Autodesk Inventor part; units mm, degrees
ref_plane "YZ Plane" through (0, 0, 0) normal (1, 0, 0) x (0, 1, 0)
ref_plane "XZ Plane" through (0, 0, 0) normal (0, 1, 0) x (-1, 0, 0)
ref_plane "XY Plane" through (0, 0, 0) normal (0, 0, 1) x (1, 0, 0)
sketch "Esquisse1" plane through (0, 0, 0) normal (0, 1, 0) x (-1, 0, 0)
  line L0 (-7, 22.5) -> (7, 22.5)
  line L1 (9, 20.5) -> (9, -20.5)
  line L2 (7, -22.5) -> (-7, -22.5)
  line L3 (-9, -20.5) -> (-9, 20.5)
  line L4 (-9, 22.5) -> (9, -22.5) construction
  line L5 (9, 22.5) -> (-9, -22.5) construction
  line L6 (-5, -17.5) -> (5, -17.5) construction
  line L7 (5, -17.5) -> (5, 17.5) construction
  line L8 (5, 17.5) -> (-5, 17.5) construction
  line L9 (-5, 17.5) -> (-5, -17.5) construction
  line L10 (-5, -17.5) -> (5, 17.5) construction
  line L11 (5, -17.5) -> (-5, 17.5) construction
  arc A0 (9, 20.5) -> (7, 22.5) centre (7, 20.5) ccw
  arc A1 (-7, 22.5) -> (-9, 20.5) centre (-7, 20.5) ccw
  arc A2 (-9, -20.5) -> (-7, -22.5) centre (-7, -20.5) ccw
  arc A3 (7, -22.5) -> (9, -20.5) centre (7, -20.5) ccw
  point P0 (0, 0)
  dimension "d0" = 18
  dimension "d1" = 45
  dimension "d3" = 4
  dimension "d4" = 5
  dimension "d25" = 2
extrude "Extrusion1" add sketch "Esquisse1" against normal blind 8
hole "Perçage1" at (-5, 0, 17.5) at (5, 0, 17.5) at (5, 0, -17.5) at (-5, 0, -17.5) direction (0, -1, 0) diameter 4.2 end through all countersink diameter 9 countersink angle 90
sketch "Esquisse2" plane through (0, 0, 0) normal (0, 1, 0) x (1, 0, 0)
  line L0 (-9, -20.5) -> (-9, 20.5) construction
  line L1 (9, 13) -> (-9, 13) construction
  line L2 (-9, 13) -> (-9, -13) construction
  line L3 (-9, -13) -> (9, -13) construction
  line L4 (9, -13) -> (9, 13) construction
  line L5 (9, 13) -> (-9, -13) construction
  line L6 (-9, 13) -> (9, -13) construction
  line L7 (9, 7.5) -> (4.2, 7.5)
  line L8 (1.2, 4.5) -> (1.2, -4.5)
  line L9 (4.2, -7.5) -> (9, -7.5)
  line L10 (9, -7.5) -> (9, 7.5)
  arc A0 (1.2, -4.5) -> (4.2, -7.5) centre (4.2, -4.5) ccw
  arc A1 (4.2, 7.5) -> (1.2, 4.5) centre (4.2, 4.5) ccw
  line L11 (9, -13) -> (-9, -13)
  line L12 (-9, -9) -> (9, -9)
  line L13 (9, -9) -> (9, -13)
  line L14 (9, 13) -> (1.2, 13)
  line L15 (1.2, 13) -> (1.2, 9)
  line L16 (1.2, 9) -> (9, 9)
  line L17 (9, 9) -> (9, 13)
  line L18 (0, -22.5) -> (0, 22.5)
  line L19 (-7, -22.5) -> (7, -22.5) construction
  line L20 (7, 22.5) -> (-7, 22.5) construction
  line L21 (-9, -13) -> (-9, 13) construction
  line L22 (-9, 7.5) -> (-4.2, 7.5)
  line L23 (-1.2, 4.5) -> (-1.2, -4.5)
  line L24 (-4.2, -7.5) -> (-9, -7.5)
  line L25 (-9, -7.5) -> (-9, 7.5)
  arc A2 (-4.2, -7.5) -> (-1.2, -4.5) centre (-4.2, -4.5) ccw
  arc A3 (-1.2, 4.5) -> (-4.2, 7.5) centre (-4.2, 4.5) ccw
  line L26 (-9, -9) -> (-9, -13)
  line L27 (-9, 13) -> (-1.2, 13)
  line L28 (-1.2, 13) -> (-1.2, 9)
  line L29 (-1.2, 9) -> (-9, 9)
  line L30 (-9, 9) -> (-9, 13)
  point P0 (0, 0)
  point P1 (-9, -22.5)
  point P2 (-9, 22.5)
  dimension "d17" = 1.5
  dimension "d19" = 15
  dimension "d20" = 4
  dimension "d21" = 3
  dimension "d22" = 4
  dimension "d23" = 1.5
  dimension "d24" = 1.2
extrude "Extrusion2" add sketch "Esquisse2" along normal blind 10
properties part number "jonction de courroie"
Check sheet for the modelled part. Datum: model origin and axes. Units: mm. A direction names the side the tool comes from. Round coordinates to 2 decimals unless told otherwise and drop trailing zeros. Order: outer loops, then holes, each group sorted by start corner. A loop starts at its lowest first (then second) coordinate and runs counter-clockwise, first axis right, second up. Notation, with made-up numbers: (26.5, 64.25) -> (58.5, 64.25) arc R14 cw to (58.5, 79.25) -> close; hole circle Ø4 at (70.25, 47). An arc over 180 degrees is marked (long way). One line per item, written item: value. Start each with the question number.
Q1. Mould release check, pull along Z, two halves, no side actions. Record for faces 6 (the face through (5, 5, -9)), 7 (the face through (0, -4, 22.5)), 8 (the face through (-8.4, -3.94, -21.93)), 9 (the face through (-2.06, 4.93, 6.6)): pulls with the +Z half, pulls with the -Z half, needs draft (parallel to the pull), parting line crosses it, or undercut.
Q2. Cross-section at B-B (y = -6.25). Record the boundary of the cut face in (x, z).
Q3. Set-up check for faces 1 (the face through (0, 5, 13)), 2 (the face through (-2.1, 4.93, -6.64)), 3 (the face through (-5, 10, -11)), 4 (the face through (7, 5, 7.5)), 5 (the face through (9, -1, 0)): record each of +Z, -Z, +X, -X, +Y, -Y from which the full face is reachable in a straight line by a thin tool's end or side.
Q4. Gauge pin test, flat ends, axial feed: pin 1 Ø2.5 at (x, y) = (7, 4.5) entering from -Z; pin 2 Ø8 at (x, y) = (4.5, 6.5) entering from +Z; pin 3 Ø0.7 at (x, z) = (7, -14) entering from +Y. Record the tip position at first contact, or that the pin passes through.
Q5. Cross-section at A-A (z = -17.5). Record the boundary of the cut face in (x, y).
Q6. Thickness scan on line 1 (X direction, y = -5.7, z = 17.5); line 2 (Z direction, x = 7, y = 0.25); line 3 (Z direction, x = -5, y = -6.5). Record the ranges inside material, lowest first.
Q7. Cross-section at D-D (z = -9.5). Record the boundary of the cut face in (x, y).
Q8. Cross-section at C-C (y = 3.75). Record the boundary of the cut face in (x, z), and give its area (3 significant figures).
Completed:
1. face 6: undercut
1. face 7: pulls with the +Z half
1. face 8: pulls with the -Z half
1. face 9: undercut
2. outline: (-9, -20.5) arc R2 ccw to (-7, -22.5) -> (7, -22.5) arc R2 ccw to (9, -20.5) -> (9, 20.5) arc R2 ccw to (7, 22.5) -> (-7, 22.5) arc R2 ccw to (-9, 20.5) -> close; hole circle Ø4.2 at (-5, -17.5); hole circle Ø4.2 at (-5, 17.5); hole circle Ø4.2 at (5, -17.5); hole circle Ø4.2 at (5, 17.5)
3. face 1: +Z, +X, -X, +Y
3. face 2: +Y
3. face 3: +Z, -Z, +X, -X, +Y
3. face 4: +X, -X, +Y
3. face 5: +Z, -Z, +X, +Y, -Y
4. pin 1: stops at z = -13
4. pin 2: stops at z = 13
4. pin 3: stops at y = -0.12
5. outline: (-9, -8) -> (-7.1, -8) -> (-7.1, -2.4) -> (-9, -0.5) -> close; (-2.9, -8) -> (2.9, -8) -> (2.9, -2.4) -> (0.5, 0) -> (-0.5, 0) -> (-2.9, -2.4) -> close; (7.1, -8) -> (9, -8) -> (9, -0.5) -> (7.1, -2.4) -> close
6. line 1: x = -9 to -7.1, -2.9 to 2.9, 7.1 to 9
6. line 2: z = -13 to -9, -7.5 to 7.5, 9 to 13
6. line 3: z = -22.5 to -19.6, -15.4 to 15.4, 19.6 to 22.5
7. outline: (-9, -8) -> (9, -8) -> (9, 10) -> (1.2, 10) -> (1.2, 0) -> (-1.2, 0) -> (-1.2, 10) -> (-9, 10) -> close
8. outline: (-9, -13) -> (-1.2, -13) -> (-1.2, -9) -> (-9, -9) -> close; (-9, -7.5) -> (-4.2, -7.5) arc R3 ccw to (-1.2, -4.5) -> (-1.2, 4.5) arc R3 ccw to (-4.2, 7.5) -> (-9, 7.5) -> close; (-9, 9) -> (9, 9) -> (9, 13) -> (-9, 13) -> close; (1.2, -13) -> (9, -13) -> (9, -9) -> (1.2, -9) -> close; (1.2, -4.5) arc R3 ccw to (4.2, -7.5) -> (9, -7.5) -> (9, 7.5) -> (4.2, 7.5) arc R3 ccw to (1.2, 4.5) -> close
8. area: 361 mm²
